Work out the finished part from the listing and answer in its coordinate system (mm). A direction names the side the tool comes from. Coordinates: 2 decimals unless noted, no trailing zeros. Order: outer loops, then holes, each group sorted by start corner. A loop starts at its lowest first (then second) coordinate and runs counter-clockwise, first axis right, second up.
1. The part is cut by section B-B, the plane y = 10. Give the vertices of the cut face in (x, z), then the cut area to 3 significant figures.
2. Find the intervals of material crossed by probe 1 along X at (y, z) = (30, 11.15); probe 2 along Y at (x, z) = (2.75, 16.25); probe 3 along X at (y, z) = (13.25, 13.5), in increasing order.
3. A tool of negligible diameter and unlimited length cuts with its end or side. For faces 4 (the flat face through (14.5, 12, 15)), 5 (the flat face through (10, 35, 15)), 6 (the flat face through (5.5, 12, 15)), 7 (the flat face through (10, 30, 13)), from which of +Z, -Z, +X, -X, +Y, -Y can it reach the whole face along a straight path? Write none if from no direction.
4. The part is cut by section A-A, the plane z = 15. Give the vertices of the cut face in (x, y).
5. Flat-ended cylindrical pins translate along their axes: pin 1 Ø4 at (x, z) = (17, 12.5) entering from -Y; pin 2 Ø2 at (y, z) = (15, 12) entering from +X. Find the tip coordinate at first contact, or state that the pin passes through.
6. The part is cut by section C-C, the plane x = 10. Give the vertices of the cut face in (y, z).
7. The part is cut by section D-D, the plane y = 30. Give the vertices of the cut face in (x, z), then the cut area to 3 significant figures.
8. Determine the mould class of faces 1 (the cylindrical face through (10.06, 8.5, 15.07)), 2 (the cylindrical face through (9.67, 27.52, 11.48)), 3 (the flat face through (1, 19, 15)) for opening direction X: +X half, -X half, draft (parallel to the pull), parting line (faces both ways), or undercut.
```python
from build123d import *

# Parameters (mm, degrees)
PAD001_DEPTH    = 10
SKETCH004_R     = 1.5
POCKET002_DEPTH = 14.501
SKETCH005_R     = 2.5
POCKET003_DEPTH = 3
FILLET_R        = 4
CHAMFER001_SIZE = 2


with BuildPart() as part:
    # Sketch003 → Pad001 (new body)
    with BuildSketch(Plane.XY):
        Polygon((0, 18), (5.5, 18), (5.5, 5.5), (14.5, 5.5), (14.5, 18), (20, 18), (20, 35), (0, 35), align=None)
    extrude(amount=PAD001_DEPTH)

    # Sketch004 (on Face4 of Pad001) → Pocket002 (cut, through all)
    with BuildSketch(Plane.YZ.offset(14.5)):
        with Locations((10, 5)):
            Circle(SKETCH004_R)
    extrude(amount=-POCKET002_DEPTH, mode=Mode.SUBTRACT)

    # Sketch005 (on Face4 of Pocket002) → Pocket003 (cut)
    with BuildSketch(Plane(origin=(0, 0, 0), x_dir=(1, 0, 0), z_dir=(0, 0, -1))):
        with Locations((10, -30)):
            Circle(SKETCH005_R)
    extrude(amount=-POCKET003_DEPTH, mode=Mode.SUBTRACT)

    # Fillet
    fillet_edges = [part.edges().sort_by_distance(p)[0] for p in [
        (10, 5.5, 10),
        (10, 5.5, 0),
    ]]
    fillet(fillet_edges, radius=FILLET_R)

    # Chamfer001
    chamfer001_edges = [part.edges().sort_by_distance(p)[0] for p in [
        (0, 35, 5),
        (0, 18, 5),
        (20, 35, 5),
        (20, 18, 5),
    ]]
    chamfer(chamfer001_edges, length=CHAMFER001_SIZE)


with BuildPart() as part_1:
    # Body001 placement: moved
    add(part.part.moved(Location((0, 0, 10))))


solid = part_1.part
```
Geometry says:
1. outline: (5.5, 10) - (14.5, 10) - (14.5, 13.5) - (5.5, 13.5) - close; (5.5, 16.5) - (14.5, 16.5) - (14.5, 20) - (5.5, 20) - close
1. area: 63.0 mm2
2. probe 1: x = 0 to 7.5, 12.5 to 20
2. probe 2: y = 18 to 35
2. probe 3: x = 5.5 to 14.5
3. face 4: +Z, -Z, +X, -Y
3. face 5: +Z, -Z, +X, -X, +Y
3. face 6: +Z, -Z, -X, -Y
3. face 7: -Z
4. outline: (0, 20) - (2, 18) - (5.5, 18) - (5.5, 11.5) - (14.5, 11.5) - (14.5, 18) - (18, 18) - (20, 20) - (20, 33) - (18, 35) - (2, 35) - (0, 33) - close; (5.5, 5.5) - (14.5, 5.5) - (14.5, 8.5) - (5.5, 8.5) - close
5. pin 1: stops at y = 18
5. pin 2: stops at x = 14.5
6. outline: (5.5, 14) arc R4 ccw to (9.5, 10) - (27.5, 10) - (27.5, 13) - (32.5, 13) - (32.5, 10) - (35, 10) - (35, 20) - (9.5, 20) arc R4 ccw to (5.5, 16) - close; hole circle Ø3 at (10, 15)
7. outline: (0, 10) - (7.5, 10) - (7.5, 13) - (12.5, 13) - (12.5, 10) - (20, 10) - (20, 20) - (0, 20) - close
7. area: 185 mm2
8. face 1: draft
8. face 2: undercut
8. face 3: -X half
